Design review of the part built by this model. Coordinates are the model's own, in mm. Round coordinates to 2 decimals unless told otherwise and drop trailing zeros. Loops run counter-clockwise (first coordinate to the right, second up) from the corner with the lowest first, then second, coordinate; pieces in that order, holes last. Notation, with made-up numbers: M 55,19.5 L 64,19.5 A26 cw 64,45.5 Z; hole C -12,88.25 d1. An arc over 180 degrees is marked long. Answer as CSV lines item,"result". Start each with the question number.
Autodesk Inventor part; units mm, degrees
ref_plane "YZ Plane" through (0, 0, 0) normal (1, 0, 0) x (0, 1, 0)
ref_plane "XZ Plane" through (0, 0, 0) normal (0, 1, 0) x (-1, 0, 0)
ref_plane "XY Plane" through (0, 0, 0) normal (0, 0, 1) x (1, 0, 0)
sketch "Sketch1" plane through (0, 0, 0) normal (1, 0, 0) x (0, 1, 0)
  line L0 (0, 0) -> (0, -609.6)
  line L1 (0, -609.6) -> (511.5151, -609.6)
  line L2 (511.5151, -609.6) -> (0, 0)
  line L3 (25.4, -69.7859) -> (457.0447, -584.2)
  line L4 (457.0447, -584.2) -> (25.4, -584.2)
  line L5 (25.4, -584.2) -> (25.4, -69.7859)
  dimension "d0" = 609.6
  dimension "d1" = 40
  dimension "d2" = 25.4
  dimension "d3" = 25.4
  dimension "d4" = 25.4
extrude "Extrusion1" add sketch "Sketch1" along normal mid plane 25.4
sketch "Sketch2" plane through (-12.7, 0, 0) normal (-1, 0, 0) x (0, 0, 1)
  line L0 (-609.6, 0) -> (-609.6, 511.5151)
  line L1 (-609.6, 511.5151) -> (0, 0)
  line L2 (-609.6, 511.5151) -> (0, 0)
  line L3 (-69.7859, 25.4) -> (-584.2, 457.0447)
  line L4 (-584.2, 457.0447) -> (-39.5154, 0)
  line L5 (0, 0) -> (-609.6, 0)
  line L6 (-584.2, 457.0447) -> (-609.6, 478.3578)
  line L7 (-609.6, 511.5151) -> (-609.6, 478.3578)
  line L8 (-39.5154, 0) -> (0, 0)
extrude "Extrusion2" add sketch "Sketch2" along normal blind 25.4 contours L0 L1 L5 L4 L3 L6
properties part number "ballRampRightSideV04"
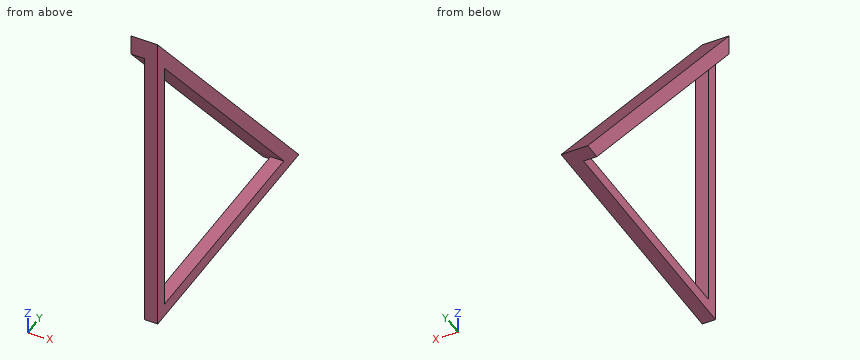
Item 1: Consider section D-D, the plane x = -30. Write out the cut boundary in (y, z).
Item 2: Consider section A-A, the plane y = 85. Write out the cut boundary in (x, z), then the cut area to 3 significant figures.
Item 3: Consider section C-C, the plane z = -391.5. Write out the cut boundary in (x, y), then the cut area to 3 significant figures.
Item 4: To check wall thickness, follow line 1 (Y direction, x = 4, z = -398); line 2 (Y direction, x = 6, z = -277.5); line 3 (Z direction, x = 4, y = 89). State the ranges of each line that lie inside material, in increasing order.
Item 5: Insertion check: pin 1 Ø7.5 at (x, z) = (-4, -409.5) entering from +Y; pin 2 Ø8 at (x, z) = (-20, -274.5) entering from +Y; pin 3 Ø4 at (x, y) = (3.5, 289.5) entering from +Z. Each pin has a flat end and moves straight along its axis. Give the tip position at first contact, or say it passes through.
Item 6: Consider section B-B, the plane x = 6. Write out the cut boundary in (y, z), then the cut area to 3 significant figures.
Found:
1,outline,"M 0,-39.52 L 457.04,-584.2 L 478.36,-609.6 L 511.52,-609.6 L 0,0 Z"
2,outline,"M -38.1,-140.81 L 12.7,-140.81 L 12.7,-101.3 L -38.1,-101.3 Z; M -12.7,-609.6 L 12.7,-609.6 L 12.7,-584.2 L -12.7,-584.2 Z"
2,area,"2,650 mm^2"
3,outline,"M -38.1,295.35 L 12.7,295.35 L 12.7,328.51 L -38.1,328.51 Z; M -12.7,0 L 12.7,0 L 12.7,25.4 L -12.7,25.4 Z"
3,area,"2,330 mm^2"
4,line 1,"y = 0 to 25.4, 300.8 to 333.96"
4,line 2,"y = 0 to 25.4, 199.69 to 232.85"
4,line 3,"z = -609.6 to -584.2, -145.58 to -106.07"
5,pin 1,"stops at y = 346.76"
5,pin 2,"stops at y = 233.69"
5,pin 3,"stops at z = -342.63"
6,outline,"M 0,-609.6 L 511.52,-609.6 L 0,0 Z; hole M 25.4,-584.2 L 457.04,-584.2 L 25.4,-69.79 Z"
6,area,"44,900 mm^2"
